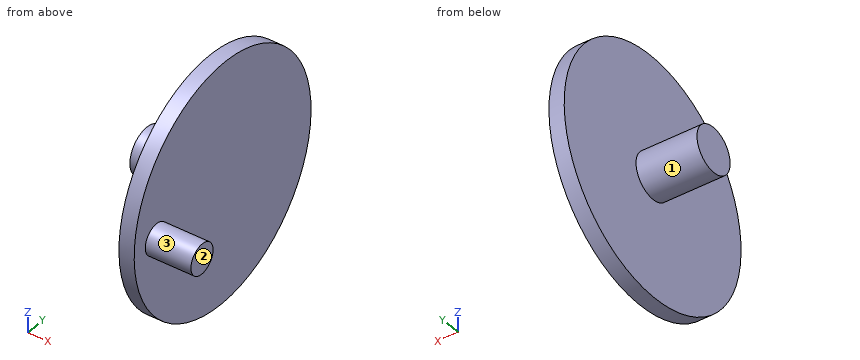
```python
from build123d import *

# Parameters (mm, degrees)
SKETCH2_R                = 7.5
BOSS_EXTRUDE1_DEPTH      = 5
BOSS_EXTRUDE1_DEPTH_BACK = 15
SKETCH3_R                = 40
BOSS_EXTRUDE2_DEPTH      = 5
SKETCH4_R                = 5
BOSS_EXTRUDE3_DEPTH      = 15


with BuildPart() as part:
    # Sketch2 → Boss-Extrude1 (new body, two sides)
    with BuildSketch(Plane(origin=(10, 0, 0), x_dir=(0, 0, -1), z_dir=(1, 0, 0))) as boss_extrude1_sk:
        with Locations((0, 60)):
            Circle(SKETCH2_R)
    extrude(amount=BOSS_EXTRUDE1_DEPTH)
    extrude(boss_extrude1_sk.sketch, amount=-BOSS_EXTRUDE1_DEPTH_BACK)

    # Sketch3 → Boss-Extrude2 (add)
    with BuildSketch(Plane(origin=(15, 0, 0), x_dir=(0, 0, -1), z_dir=(1, 0, 0))):
        with Locations((0, 60)):
            Circle(SKETCH3_R)
    extrude(amount=BOSS_EXTRUDE2_DEPTH)

    # Sketch4 → Boss-Extrude3 (add)
    with BuildSketch(Plane(origin=(20, 0, 0), x_dir=(0, 0, -1), z_dir=(1, 0, 0))):
        with Locations((0, 30)):
            Circle(SKETCH4_R)
    extrude(amount=BOSS_EXTRUDE3_DEPTH)


solid = part.part
```
Could you check a few things on this model? Use its own coordinates, in mm. Face numbers are marked on the shaded views. A direction names the side the tool comes from. Coordinates: 2 decimals unless noted, no trailing zeros. Loops run counter-clockwise (first coordinate to the right, second up) from the corner with the lowest first, then second, coordinate; pieces in that order, holes last. Notation, with made-up numbers: M 70,10 L 108,10 A9 ccw 108,26 Z; hole C 37.25,17.25 d8. An arc over 180 degrees is marked long. Put each result on its own line as item: value. Start each with the question number.
(1) Will these pins go through, and if not, where does the flat tip stop? P1, Ø10, axis at x = 18, y = 35, coming from the +Z side; P2, Ø10, axis at x = 0.5, y = 68, coming from the -Z side; P3, Ø10, axis at x = 19, z = 24.5, coming from the -Y side.
(2) Suppose I cut it at D-D on y = 30. Please give me the cut outline in (x, z).
(3) Suppose I cut it at B-B on z = 0. Please give me the cut outline in (x, y), then the cut area to 3 significant figures.
(4) For the marked faces 1, 2 and 3, which set-ups out of +Z, -Z, +X, -X, +Y, -Y let a thin tool reach every point of the face, with its end or its side?
(5) Suppose I cut it at A-A on y = 60. Please give me the cut outline in (x, z).
(6) I need wall thicknesses on line 1 (X direction, y = 33.5, z = 1.5); line 2 (X direction, y = 82, z = 32); line 3 (Z direction, x = 19.5, y = 61). Which ranges of each line are inside material? Lowest first, please. Write a range as from..to.
(7) Suppose I cut it at C-C on x = 14. Please give me the cut outline in (y, z), then the cut area to 3 significant figures.
Solutions:
1. P1: stops at z = 34.64
1. P2: stops at z = -6.87
1. P3: stops at y = 25.08
2. outline: M 15,-26.46 L 20,-26.46 L 20,-5 L 35,-5 L 35,5 L 20,5 L 20,26.46 L 15,26.46 Z
3. outline: M -5,52.5 L 15,52.5 L 15,20 L 20,20 L 20,25 L 35,25 L 35,35 L 20,35 L 20,100 L 15,100 L 15,67.5 L -5,67.5 Z
3. area: 850 mm2
4. face 1: -X
4. face 2: +Z, -Z, +X, +Y, -Y
4. face 3: +X
5. outline: M -5,-7.5 L 15,-7.5 L 15,-40 L 20,-40 L 20,40 L 15,40 L 15,7.5 L -5,7.5 Z
6. line 1: x = 15..35
6. line 2: x = 15..20
6. line 3: z = -39.99..39.99
7. outline: C 60,0 d15
7. area: 177 mm2
